Design review of the part shown in the three views and the two pictorial views. Dimensions are in mm from the part's minimum x, y and z. A direction names the side the tool comes from. Give positions to 0.01 mm unless a question says otherwise; leave off trailing zeros. Loops run counter-clockwise (first coordinate to the right, second up) from the corner with the lowest first, then second, coordinate; pieces in that order, holes last.
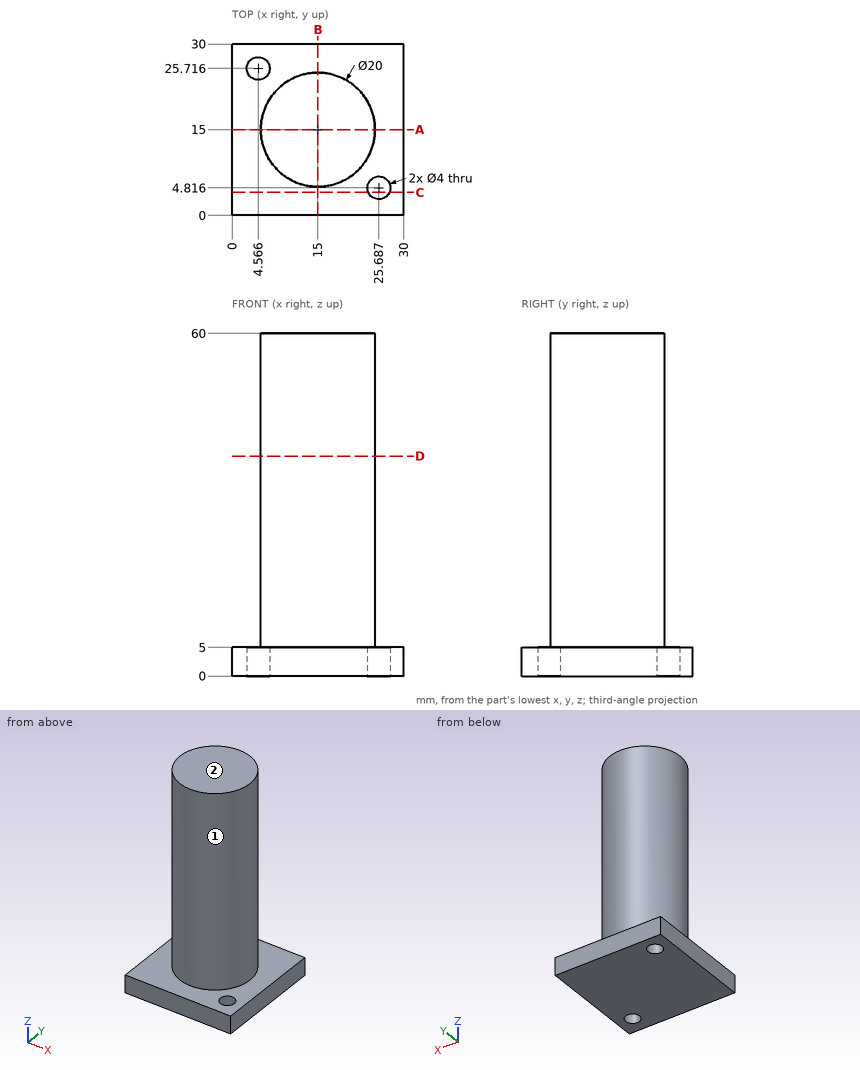
Q1. Consider section C-C on y = 4. Give the boundary of the cut face in (x, z).
Answers:
outline: (0, 0) - (23.86, 0) - (23.86, 5) - (0, 5) - close; (27.51, 0) - (30, 0) - (30, 5) - (27.51, 5) - close
Q2. For probe 1 along Z at (x, y) = (24.25, 7); probe 2 along X at (y, z) = (15.5, 54), list the stretches that pass through material, from the lowest coordinate up.
Answers:
probe 1: z = 0 to 5
probe 2: x = 5.01 to 24.99
Q3. For pin 1 Ø10 at (y, z) = (25, 47) entering from +X; pin 2 Ø8 at (x, z) = (6.5, 18) entering from -Y; pin 3 Ø3 at (x, y) = (16.5, 26.5) entering from -Z; pin 4 Ø8 at (x, z) = (10, 28.5) entering from +Y, all flat-tipped, find the tip position at first contact; note any pin that passes through.
Answers:
pin 1: stops at x = 23.66
pin 2: stops at y = 6.07
pin 3: stops at z = 0
pin 4: stops at y = 24.95
Q4. Machinability: for the marked faces 1 and 2, which of the approach directions +Z, -Z, +X, -X, +Y, -Y give a long, thin tool a straight path to every point of the face, cutting with its end or side? Answer none if there is none.
Answers:
face 1: +Z
face 2: +Z, +X, -X, +Y, -Y
Q5. Consider section D-D on z = 38.5. Give the boundary of the cut face in (x, y), plus the area to 3 significant figures.
Answers:
outline: circle Ø20 at (15, 15)
area: 314 mm2
Q6. Consider section A-A on y = 15. Give the boundary of the cut face in (x, z), plus the area to 3 significant figures.
Answers:
outline: (0, 0) - (30, 0) - (30, 5) - (25, 5) - (25, 60) - (5, 60) - (5, 5) - (0, 5) - close
area: 1,250 mm2
